Study the drawing (mm; zero at the part's minimum x, y, z) and answer. A direction names the side the tool comes from. Round coordinates to 2 decimals unless told otherwise and drop trailing zeros. Loops run counter-clockwise (first coordinate to the right, second up) from the corner with the lowest first, then second, coordinate; pieces in that order, holes last. Notation, with made-up numbers: (76, 71.25) - (91, 71.25) arc R26 ccw to (91, 97.25) - close; hole circle Ø3 at (-19, 23). An arc over 180 degrees is marked (long way). Use CSV: the item, a comma, the result in double quotes. Start each with the question number.
1. Find section A-A (x = 58). Give the vertices of the cut face in (y, z).
2. A tool of negligible diameter and unlimited length cuts with its end or side. For the marked faces 1, 2 and 3, from which of +Z, -Z, +X, -X, +Y, -Y can it reach the whole face along a straight path? Write none if from no direction.
3. Find section B-B (z = 60). Give the vertices of the cut face in (x, y), and give its area (3 significant figures).
4. Find section D-D (z = 109). Give the vertices of the cut face in (x, y), and give its area (3 significant figures).
5. Determine the mould class of the marked faces 4, 5 and 6 for opening direction X: +X half, -X half, draft (parallel to the pull), parting line (faces both ways), or undercut.
6. Consider line 1 along X through (y, z) = (1.9, 60); line 2 along Z through (x, y) = (6, 2.3); line 3 along X through (y, z) = (15, 58.5). Determine where each line is inside the solid, lowest interval first.
7. Find section C-C (y = 14.5). Give the vertices of the cut face in (x, z).
8. Given pin 1 Ø1 at (y, z) = (5, 102.5) entering from +X; pin 2 Ø10 at (x, z) = (49.5, 25) entering from +Y; pin 3 Ø2 at (x, z) = (23.5, 39) entering from -Y, each flat-ended and moving along its own axis, determine where each tip first touches the part or whether it passes through.
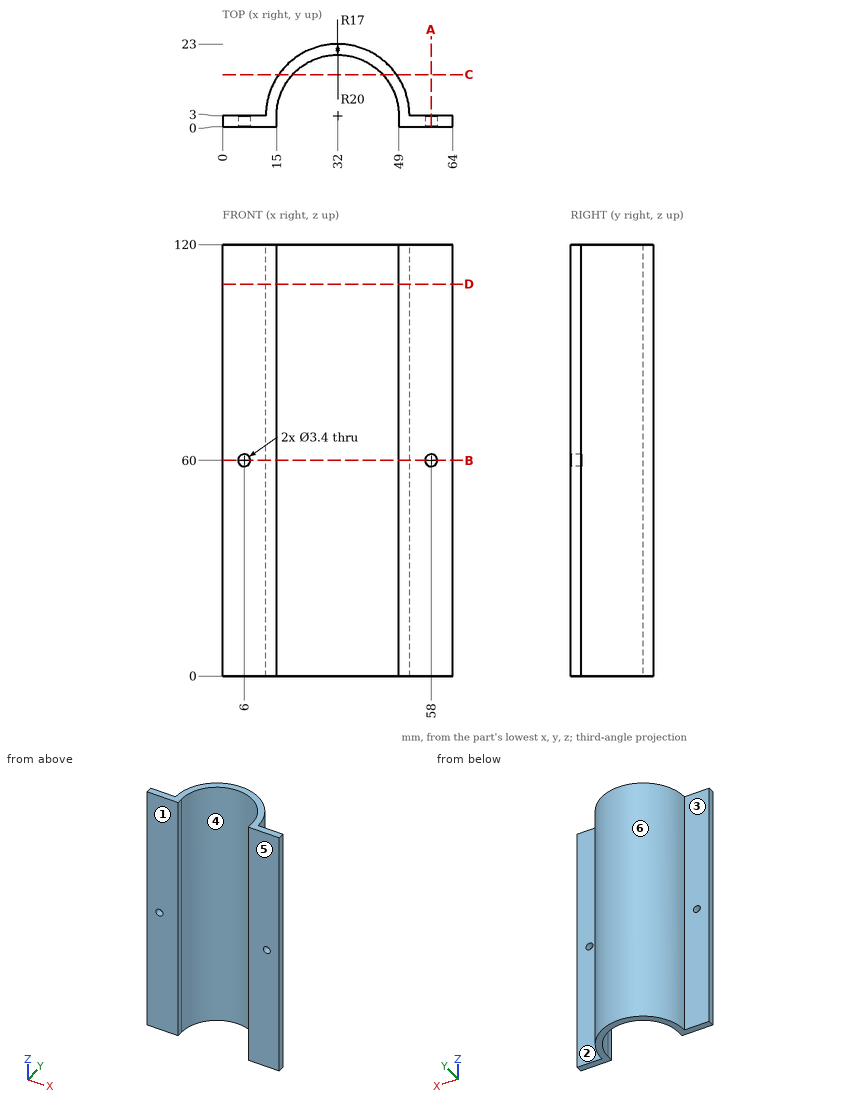
Filled sheet:
1,outline,"(0, 0) - (3, 0) - (3, 58.3) - (0, 58.3) - close; (0, 61.7) - (3, 61.7) - (3, 120) - (0, 120) - close"
2,face 1,"+Z, -Z, +X, -X, -Y"
2,face 2,"+Z, -Z, +X, +Y"
2,face 3,"+Z, -Z, -X, +Y"
3,outline,"(0, 0) - (4.3, 0) - (4.3, 3) - (0, 3) - close; (7.7, 0) - (15, 0) - (15, 3) arc R17 cw to (49, 3) - (49, 0) - (56.3, 0) - (56.3, 3) - (52, 3) arc R20 ccw to (12, 3) - (7.7, 3) - close; (59.7, 0) - (64, 0) - (64, 3) - (59.7, 3) - close"
3,area,"244 mm²"
4,outline,"(0, 0) - (15, 0) - (15, 3) arc R17 cw to (49, 3) - (49, 0) - (64, 0) - (64, 3) - (52, 3) arc R20 ccw to (12, 3) - (0, 3) - close"
4,area,"264 mm²"
5,face 4,"undercut"
5,face 5,"draft"
5,face 6,"parting line"
6,line 1,"x = 0 to 4.3, 7.7 to 15, 49 to 56.3, 59.7 to 64"
6,line 2,"z = 0 to 58.3, 61.7 to 120"
6,line 3,"x = 16 to 19.96, 44.04 to 48"
7,outline,"(15.64, 0) - (19.48, 0) - (19.48, 120) - (15.64, 120) - close; (44.52, 0) - (48.36, 0) - (48.36, 120) - (44.52, 120) - close"
8,pin 1,"stops at x = 51.94"
8,pin 2,"stops at y = 18.61"
8,pin 3,"stops at y = 17.1"
